from build123d import *

# Parameters (mm, degrees)
PAD_DEPTH   = 50
THICKNESS_T = 1.5


with BuildPart() as part:
    # Sketch → Pad (new body)
    with BuildSketch(Plane.XY):
        with BuildLine():
            ThreePointArc((3, 0), (0.87868, -0.87868), (0, -3))
            Line((0, -107), (0, -3))
            ThreePointArc((0, -107), (0.87868, -109.12132), (3, -110))
            Line((75, -110), (3, -110))
            ThreePointArc((75, -110), (77.12132, -109.12132), (78, -107))
            Line((78, -3), (78, -107))
            ThreePointArc((78, -3), (77.12132, -0.87868), (75, 0))
            Line((3, 0), (75, 0))
        make_face()
    extrude(amount=PAD_DEPTH)

    # Thickness
    thickness_openings = [part.faces().sort_by_distance(p)[0] for p in [
        (39, -55, 50),
    ]]
    offset(amount=THICKNESS_T, openings=thickness_openings)


solid = part.part
Work out the finished part from the listing and answer in its coordinate system (mm). A direction names the side the tool comes from. Coordinates: 2 decimals unless noted, no trailing zeros. Loops run counter-clockwise (first coordinate to the right, second up) from the corner with the lowest first, then second, coordinate; pieces in that order, holes last. Notation, with made-up numbers: (-6.75, 8) -> (-0.75, 8) arc R17 cw to (-0.75, 33) -> close; hole circle Ø6 at (31.25, 3). An arc over 180 degrees is marked (long way). Write each question's results on one line, items separated by ' | '. Start each with the question number.
1) Find section A-A on z = 22. Determine the outline of the cut face in (x, y).
2) A flat-ended cylindrical pin translates along its axis: P1, Ø12, axis at x = 45.5, y = -99.5, coming from the +Z side. Find the tip coordinate at first contact, or state that the pin passes through.
3) For faces 4 (the cylindrical face through (77.1, -109.14, 24.65)), 5 (the cylindrical face through (78.147, -110.217, 24.65)), determine the directions among +Z, -Z, +X, -X, +Y, -Y from which every point of the face is accessible in a straight line to the end or side of a thin tool.
4) Consider line 1 along X through (y, z) = (-3, 17); line 2 along Y through (x, z) = (55, 19); line 3 along Z through (x, y) = (38, -79). Determine where each line is inside the solid, lowest interval first.
5) Find section B-B on y = -99. Determine the outline of the cut face in (x, z), then the cut area to 3 significant figures.
6) Find section C-C on x = 63. Determine the outline of the cut face in (y, z).
7) The mould has two halves that part along Y. Classify faces 1 (the cylindrical face through (-0.147, 0.217, 24.65)), 2 (the cylindrical face through (77.14, -0.9, 24.65)), 3 (the flat face through (-0.2, -54.7, 50)): pulls with the +Y half, pulls with the -Y half, needs draft (parallel to the pull), parting line crosses it, or undercut.
Response values:
1) outline: (-1.5, -107) arc R4.5 ccw to (3, -111.5) -> (75, -111.5) arc R4.5 ccw to (79.5, -107) -> (79.5, -3) arc R4.5 ccw to (75, 1.5) -> (3, 1.5) arc R4.5 ccw to (-1.5, -3) -> close; hole (0, -107) arc R3 ccw to (3, -110) -> (75, -110) arc R3 ccw to (78, -107) -> (78, -3) arc R3 ccw to (75, 0) -> (3, 0) arc R3 ccw to (0, -3) -> close
2) P1: stops at z = 0
3) face 4: +Z | face 5: +Z, -Z, +X, -Y
4) line 1: x = -1.5 to 0, 78 to 79.5 | line 2: y = -111.5 to -110, 0 to 1.5 | line 3: z = -1.5 to 0
5) outline: (-1.5, 0) arc R1.5 ccw to (0, -1.5) -> (78, -1.5) arc R1.5 ccw to (79.5, 0) -> (79.5, 50) -> (78, 50) -> (78, 0) -> (0, 0) -> (0, 50) -> (-1.5, 50) -> close | area: 271 mm^2
6) outline: (-111.5, 0) arc R1.5 ccw to (-110, -1.5) -> (0, -1.5) arc R1.5 ccw to (1.5, 0) -> (1.5, 50) -> (0, 50) -> (0, 0) -> (-110, 0) -> (-110, 50) -> (-111.5, 50) -> close
7) face 1: pulls with the +Y half | face 2: undercut | face 3: needs draft
